Answer from the drawing. Dimensions are ordinates in mm from the lowest x, y and z of the part. A direction names the side the tool comes from. Coordinates: 2 decimals unless noted, no trailing zeros. Order: outer loops, then holes, each group sorted by start corner. A loop starts at its lowest first (then second) coordinate and runs counter-clockwise, first axis right, second up. Notation, with made-up numbers: (-11, -5) - (19, -5) arc R27 ccw to (19, 24) - close; hole circle Ø10 at (-6.5, -23.75). An arc over 180 degrees is marked (long way). Answer as a JSON object with one key per item and string values. Group by question number.
1) Each of these flat-tipped pins is pushed along its axis until it touches: P1, Ø1.5, axis at x = 4, y = 11.5, coming from the +Z side; P2, Ø5, axis at x = 2.5, z = 37, coming from the -Y side; P3, Ø5, axis at y = 30, z = 50, coming from the +X side; P4, Ø4, axis at x = 5.5, z = 12.5, coming from the -Y side. Where does it stop, or does it pass through?
2) Section D-D (z = 50) is taken. Give the vertices of the cut face in (x, y).
3) Section B-B (z = 30) is taken. Give the vertices of the cut face in (x, y).
4) Section C-C (y = 30) is taken. Give the vertices of the cut face in (x, z), plus the area to 3 significant figures.
5) A tool of negligible diameter and unlimited length cuts with its end or side. For the marked faces 1 and 2, from which of +Z, -Z, +X, -X, +Y, -Y can it reach the whole face along a straight path? Write none if from no direction.
6) Find the intervals of material crossed by line 1 along Z through (x, y) = (2, 50); line 2 along Z through (x, y) = (6.25, 10); line 3 along Y through (x, z) = (0.75, 8.5), in increasing order.
7) Section A-A (x = 1.5) is taken. Give the vertices of the cut face in (y, z).
8) The mould has two halves that part along Z. Classify the marked faces 3, 4 and 5: released by +Z, released by -Z, zero draft, split by the parting line, or undercut.
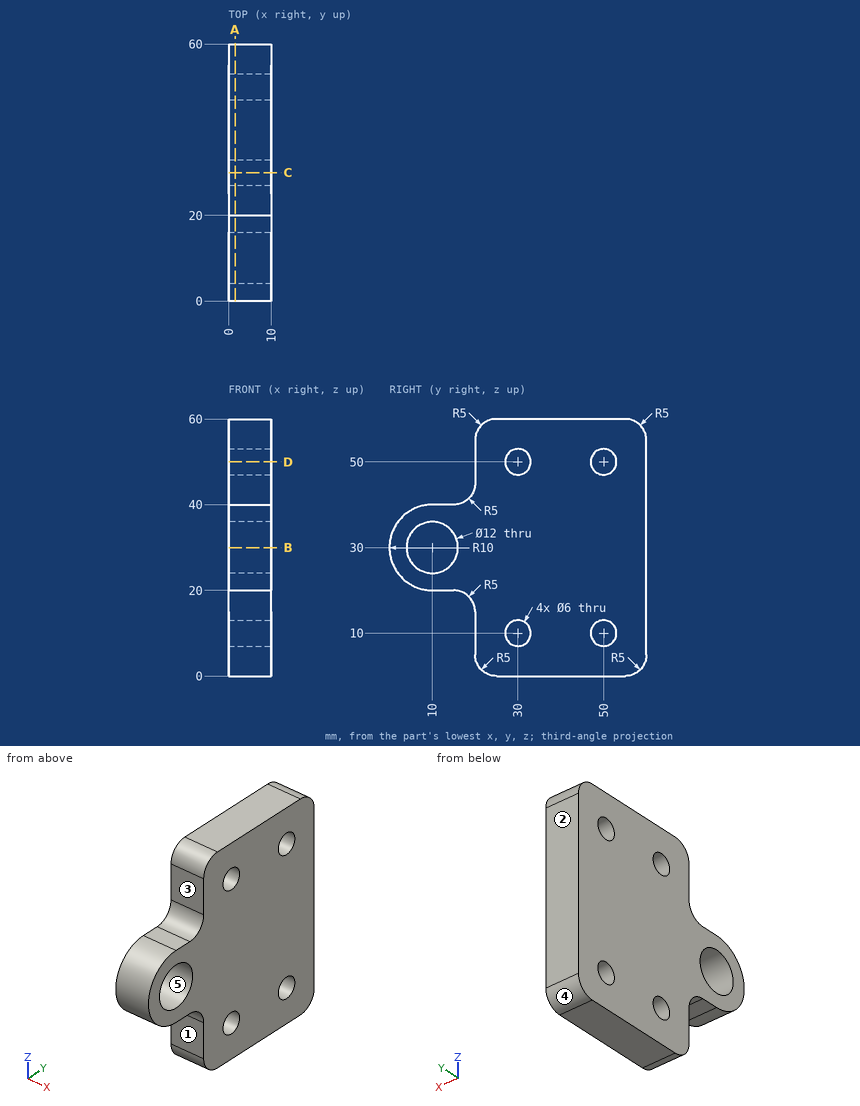
Report:
{
 "1": {"P1": "stops at z = 40", "P2": "stops at y = 1.07", "P3": "passes through", "P4": "stops at y = 20"},
 "2": {"outline": "(0, 20) - (10, 20) - (10, 27) - (0, 27) - close; (0, 33) - (10, 33) - (10, 47) - (0, 47) - close; (0, 53) - (10, 53) - (10, 60) - (0, 60) - close"},
 "3": {"outline": "(0, 0) - (10, 0) - (10, 4) - (0, 4) - close; (0, 16) - (10, 16) - (10, 60) - (0, 60) - close"},
 "4": {"outline": "(0, 0) - (10, 0) - (10, 7) - (0, 7) - close; (0, 13) - (10, 13) - (10, 47) - (0, 47) - close; (0, 53) - (10, 53) - (10, 60) - (0, 60) - close", "area": "480 mm²"},
 "5": {"face 1": "-Z, +X, -X, -Y", "face 2": "+Z, -Z, +X, -X, +Y"},
 "6": {"line 1": "z = 0 to 7, 13 to 47, 53 to 60", "line 2": "z = 20 to 24, 36 to 40", "line 3": "y = 20 to 27.4, 32.6 to 47.4, 52.6 to 60"},
 "7": {"outline": "(10, 20) - (15, 20) arc R5 cw to (20, 15) - (20, 5) arc R5 ccw to (25, 0) - (55, 0) arc R5 ccw to (60, 5) - (60, 55) arc R5 ccw to (55, 60) - (25, 60) arc R5 ccw to (20, 55) - (20, 45) arc R5 cw to (15, 40) - (10, 40) arc R10 ccw to start; hole circle Ø12 at (10, 30); hole circle Ø6 at (30, 10); hole circle Ø6 at (30, 50); hole circle Ø6 at (50, 10); hole circle Ø6 at (50, 50)"},
 "8": {"face 3": "zero draft", "face 4": "released by -Z", "face 5": "undercut"}
}
